Can you work these out from the model? Positions are in its coordinate system, mm. Face numbers are marked on the shaded views. Coordinates: 2 decimals unless noted, no trailing zeros. Write each loop counter-clockwise with the first axis right and the second up, starting at its lowest first coordinate (ties: lowest second). Pieces come first, ordered by that corner, then holes. Notation, with made-up numbers: (43, -35.5) - (77, -35.5) arc R33 cw to (77, -7.5) - close; hole circle Ø1 at (49, 50). An arc over 180 degrees is marked (long way). Write each question's results on one line, items separated by ' | '. Start each with the question number.
Autodesk Inventor part; units mm, degrees
ref_plane "YZ Plane" through (0, 0, 0) normal (1, 0, 0) x (0, 1, 0)
ref_plane "XZ Plane" through (0, 0, 0) normal (0, 1, 0) x (-1, 0, 0)
ref_plane "XY Plane" through (0, 0, 0) normal (0, 0, 1) x (1, 0, 0)
sketch "Sketch1" plane through (0, 0, 0) normal (0, 1, 0) x (-1, 0, 0)
  line L0 (-6.364, 4.3033) -> (-6.364, 17.3033)
  line L1 (-6.364, 4.3033) -> (-6.364, -8.6967)
  line L2 (-6.364, 17.3033) -> (-6.364, 20.3033)
  line L3 (-3.6569, 19.6569) -> (-26.2843, 42.2843)
  line L4 (-26.2843, 42.2843) -> (-27.6985, 40.8701)
  line L5 (-3.6569, -9.3431) -> (-3.6569, -12.3431)
  line L6 (-3.6569, -12.3431) -> (-26.2843, -34.9706)
  line L7 (-26.2843, -34.9706) -> (-28.2843, -32.9706)
  line L8 (-28.2843, -32.9706) -> (-6.364, -11.0503)
  line L9 (-6.364, -11.0503) -> (-6.364, -8.6967)
  line L10 (-3.6569, 19.6569) -> (-3.6569, -12.3431)
  line L11 (-3.6569, -12.3431) -> (-26.2843, -34.9706)
  line L12 (-28.2843, -32.9706) -> (-26.2843, -34.9706)
  line L13 (-28.2843, -32.9706) -> (-6.364, -11.0503)
  line L14 (-6.364, -11.0503) -> (-6.364, 19.5355)
  line L15 (-27.6985, 40.8701) -> (-26.2843, 42.2843)
  line L16 (-26.2843, 42.2843) -> (-3.6569, 19.6569)
  line L17 (-3.6569, 19.6569) -> (-0.6568, 19.6569) construction
  line L18 (-6.364, 18.3639) -> (-28.2843, 40.2842) construction
  line L19 (-28.2843, 40.2842) -> (-26.2843, 42.2843) construction
  line L20 (-26.2843, 42.2843) -> (-28.2843, 40.2842)
  line L21 (-6.364, 18.3639) -> (-28.2843, 40.2842)
  point P0 (0, 0)
  dimension "d64" = 32
  dimension "d65" = 32
  dimension "d66" = 2
  dimension "d67" = 32
  dimension "d70" = 31
extrude "Extrusion2" add sketch "Sketch1" along normal blind 8
sketch "Sketch9" plane through (3.6569, 0, -12.3431) normal (-1, 0, 0) x (0, 0, 1)
  line L0 (0, 0) -> (0, 8)
  line L1 (0, 8) -> (32, 8)
  line L2 (0, 8) -> (32, 8)
  line L3 (0, 8) -> (16, 8)
  line L4 (16, 8) -> (32, 8)
  line L5 (16, 8) -> (16, 0)
  line L6 (16, 0) -> (3, 0)
  line L7 (30.707, 0) -> (1.2929, 0)
  line L8 (3, 0) -> (6, 0)
  line L9 (6, 0) -> (6, 5)
  line L10 (6, 5) -> (16, 5)
  line L11 (16, 5) -> (26, 5)
  line L12 (26, 5) -> (26, 0)
  circle A0 centre (6, 5) radius 1.525
  circle A1 centre (26, 5) radius 1.525
  point P0 (12.3431, 0)
  dimension "d72" = 16
  dimension "d73" = 13
  dimension "d74" = 3
  dimension "d75" = 5
  dimension "d76" = 10
  dimension "d77" = 3.05
  dimension "d78" = 3.05
extrude "Extrusion7" cut sketch "Sketch9" against normal blind 8 contours A0 L9 L10 | L10 L9 A0 | A1 L12 L11 | L11 L12 A1
sketch "Sketch10" plane through (3.6569, 0, -12.3431) normal (-0.7071, 0, -0.7071) x (-0.7071, 0, 0.7071)
  line L0 (-32, 0) -> (0, 0)
  line L1 (-16, 0) -> (-32, 0)
  line L2 (-32, 0) -> (-16, 0)
  line L3 (0, 0) -> (-16, 0)
  line L4 (-16, 0) -> (-29, 0)
  line L5 (-29, 0) -> (-26, 0)
  line L6 (-26, 0) -> (-26, 5)
  line L7 (-26, 5) -> (-16, 5)
  line L8 (-16, 5) -> (-6, 5)
  line L9 (-6, 5) -> (-6, 0)
  circle A0 centre (-26, 5) radius 1.525
  circle A1 centre (-6, 5) radius 1.525
  point P0 (11.3137, 0)
  dimension "d81" = 13
  dimension "d82" = 3
  dimension "d83" = 5
  dimension "d84" = 10
  dimension "d85" = 3.05
  dimension "d86" = 3.05
extrude "Extrusion8" cut sketch "Sketch10" against normal blind 8 contours A0 L7 L6 | L6 L7 A0 | A1 L8 L9 | L9 L8 A1
sketch "Sketch11" plane through (26.2843, 0, 42.2843) normal (-0.7071, 0, 0.7071) x (0.7071, 0, 0.7071)
  line L0 (-32, 0) -> (-32, 8)
  line L1 (-32, 0) -> (0, 0)
  line L2 (-32, 0) -> (0, 0)
  line L3 (0, 0) -> (-16, 0)
  line L4 (-16, 0) -> (-32, 0)
  line L5 (-16, 0) -> (-29, 0)
  line L6 (0, 0) -> (-31.0001, 0)
  line L7 (-29, 0) -> (-26, 0)
  line L8 (-26, 0) -> (-26, 5)
  line L9 (-26, 5) -> (-16, 5)
  line L10 (-16, 5) -> (-6, 5)
  line L11 (-6, 5) -> (-6, 0)
  circle A0 centre (-26, 5) radius 1.525
  circle A1 centre (-6, 5) radius 1.525
  point P0 (-48.4853, 0)
  dimension "d89" = 16
  dimension "d90" = 13
  dimension "d91" = 3
  dimension "d92" = 5
  dimension "d93" = 10
  dimension "d94" = 3.05
  dimension "d95" = 3.05
extrude "Extrusion9" cut sketch "Sketch11" against normal blind 8 contours A0 L9 L8 | L8 L9 A0 | A1 L10 L11 | L11 L10 A1
sketch "Sketch12" plane through (0, 0, 0) normal (0, -1, 0) x (1, 0, 0)
  line L0 (3.6569, -12.3431) -> (3.6569, 19.6569)
  line L1 (3.6569, -12.3431) -> (3.6569, 19.6569)
  line L2 (3.6569, 19.6569) -> (3.6569, 3.6569)
  line L3 (3.6569, 3.6569) -> (6.364, 3.6568)
  line L4 (6.364, 18.3639) -> (6.364, -11.0503)
  point P0 (0, 0)
  dimension "d98" = 16
properties part number "distanceSensorMount"
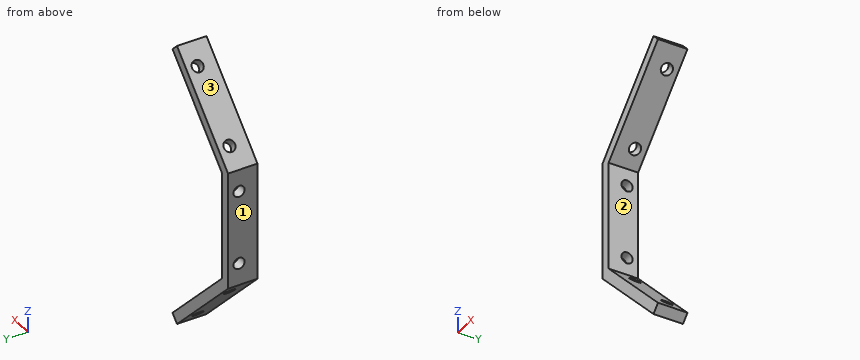
Q1. If we section it at A-A (y = 5): Count the separate pieces of the cut face and the enclosed holes in it, then the cut area to 3 significant figures.
Q2. I need wall thicknesses on line 1 along Z through (x, y) = (5.75, 5); line 2 along Z through (x, y) = (4.9, 5); line 3 along X through (y, z) = (1.25, 16). Which ranges of each line are inside material? Lowest first, please. Write a range as from..to.
Q3. If we section it at B-B (z = -1.5): Please give me the cut outline in (x, y), then the cut area to 3 significant figures.
Q4. I'm going to push flat-ended pins straight in: pin 1 Ø1.8 at (y, z) = (5, -6.34) entering from +X; pin 2 Ø3 at (x, y) = (21.5, 6) entering from +Z; pin 3 Ø2 at (y, z) = (4, -5.5) entering from +X; pin 4 Ø2 at (x, y) = (9, 3.5) entering from -Z. Where does each tip first touch, or does it pass through?
Q5. Thinking about a two-plate mould opening in Z: for the marked faces 1, 2 and 3, which applies, pulls with the +Z half, pulls with the -Z half, needs draft (parallel to the pull), parting line crosses it, or undercut?
Q6. If we section it at C-C (y = 1.75): Please give me the cut outline in (x, z).
Answer list:
1) separate pieces: 7 | enclosed holes: 0 | area: 210 mm2
2) line 1: z = -14.44..-7.87, -4.82..12.13, 15.18..21.75 | line 2: z = -13.59..-7.87, -4.82..12.13, 15.18..20.9 | line 3: x = 3.66..6.36
3) outline: (3.66, 0) - (6.36, 0) - (6.36, 8) - (3.66, 8) - close | area: 21.7 mm2
4) pin 1: passes through | pin 2: stops at z = 39 | pin 3: stops at x = 6.36 | pin 4: stops at z = -18.69
5) face 1: needs draft | face 2: undercut | face 3: pulls with the +Z half
6) outline: (3.66, -12.34) - (26.28, -34.97) - (28.28, -32.97) - (6.36, -11.05) - (6.36, 18.36) - (28.28, 40.28) - (27.7, 40.87) - (26.28, 42.28) - (3.66, 19.66) - close
